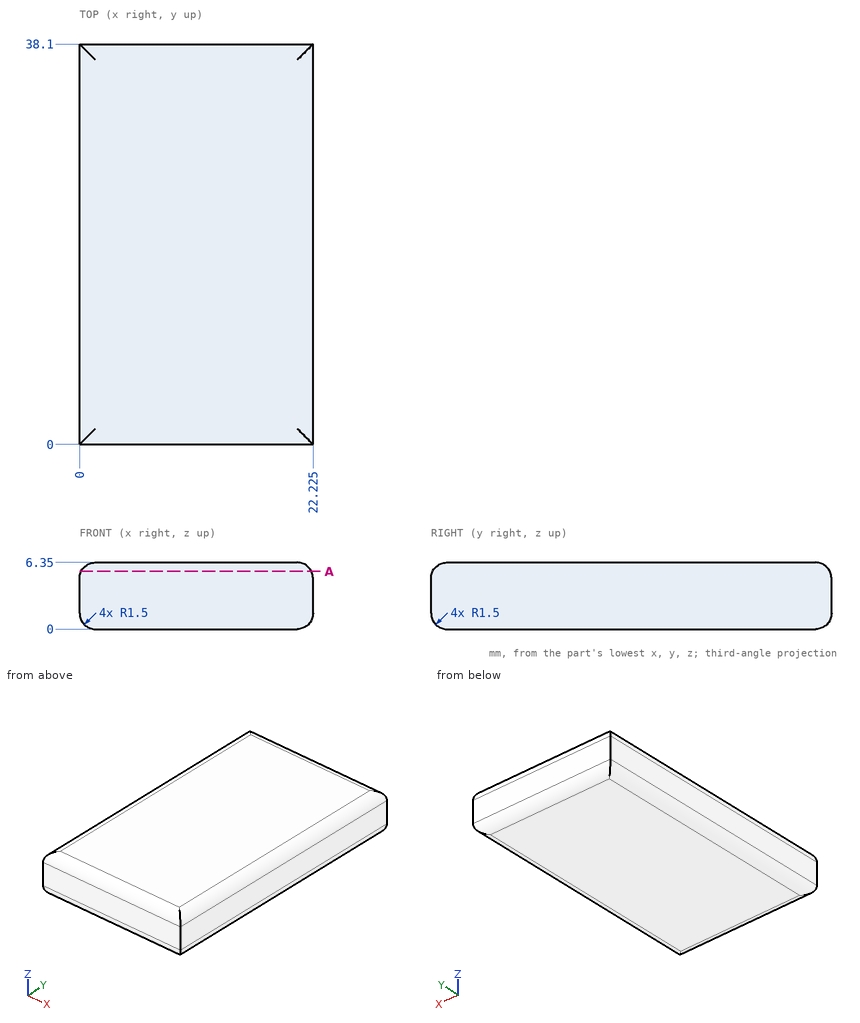
Drawing for the job (mm, zero at the part's lowest x, y, z). Coordinates: 2 decimals unless noted, no trailing zeros. Write each loop counter-clockwise with the first axis right and the second up, starting at its lowest first coordinate (ties: lowest second). Pieces come first, ordered by that corner, then holes. Notation, with made-up numbers: (-29, 87) -> (23, 87) arc R22 ccw to (23, 124) -> close; hole circle Ø9 at (35.5, 55.25). An arc over 180 degrees is marked (long way). One line per item, written item: value. Start each with the question number.
1) Slice it at A-A on z = 5.5. Write the cut outline in (x, y).
2) Probe probe 1 along Y at (x, z) = (6.75, 5); probe 2 along X at (y, z) = (25, 5); probe 3 along X at (y, z) = (11, 1). List the from-to ranges inside material, lowest first.
3) Flat gauge pin, fed straight in: pin 1 Ø8 at (x, y) = (8, 13) entering from -Z. Where does the tip first touch, or does it go through?
Answers follow:
1. outline: (0.15, 0.15) -> (22.08, 0.15) -> (22.08, 37.95) -> (0.15, 37.95) -> close
2. probe 1: 0.01 to 38.09
2. probe 2: 0.01 to 22.22
2. probe 3: 0.09 to 22.14
3. pin 1: z = 0
